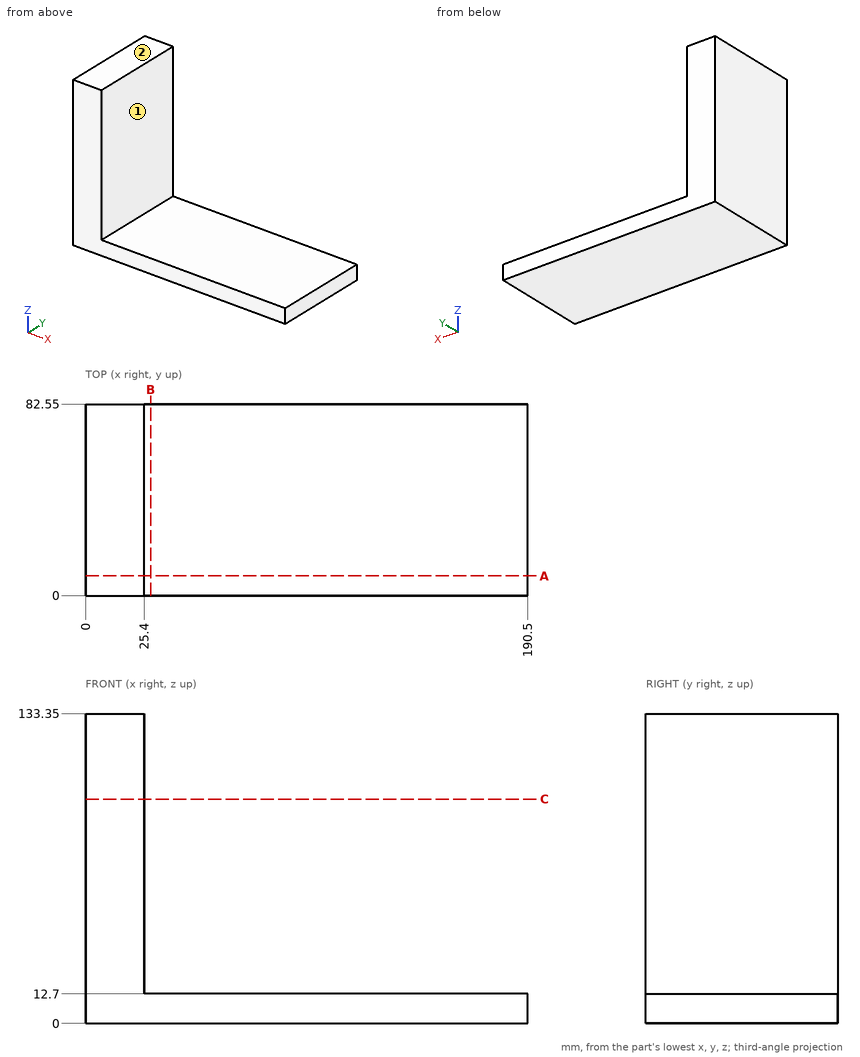
For this review, use the dimensioned drawing (mm, ordinates from the lowest corner) and the shaded views. A direction names the side the tool comes from. Give positions to 0.01 mm unless a question says otherwise; leave off trailing zeros. Write each loop counter-clockwise with the first axis right and the second up, starting at its lowest first coordinate (ties: lowest second). Pieces come first, ordered by that corner, then holes. Notation, with made-up numbers: M -1.5,58.25 L 17.5,58.25 A21 ccw 17.5,78.25 Z; hole C 9.25,-13 d6. An arc over 180 degrees is marked long. Write item = value, one per line. Start each with the question number.
Q1. We need section A-A (y = 8.5). State the section outline as (x, z) points, plus the area to 3 significant figures.
Q2. We need section B-B (x = 28). State the section outline as (y, z) points, plus the area to 3 significant figures.
Q3. Clearance check with a flat-ended pin moving along its axis: pin 1 (4 mm diameter, centred on x = 142.5, y = 35.5, fed in from +Z). State where the tip first meets the part, or that it passes through.
Q4. For line 1 (Z direction, x = 158.5, y = 67); line 2 (X direction, y = 38, z = 81.5), list the stretches that pass through material, from the lowest coordinate up.
Q5. Machinability: for the marked faces 1 and 2, which of the approach directions +Z, -Z, +X, -X, +Y, -Y give a long, thin tool a straight path to every point of the face, cutting with its end or side? Answer none if there is none.
Q6. We need section C-C (z = 96.5). State the section outline as (x, y) points.
Result set:
q1.outline = M 0,0 L 190.5,0 L 190.5,12.7 L 25.4,12.7 L 25.4,133.35 L 0,133.35 Z
q1.area = 5,480 mm2
q2.outline = M 0,0 L 82.55,0 L 82.55,12.7 L 0,12.7 Z
q2.area = 1,050 mm2
q3.pin_1 = 12.7
q4.line_1 = 0 to 12.7
q4.line_2 = 0 to 25.4
q5.face_1 = +Z, +X, +Y, -Y
q5.face_2 = +Z, +X, -X, +Y, -Y
q6.outline = M 0,0 L 25.4,0 L 25.4,82.55 L 0,82.55 Z
